Job drawing, mm, ordinate dimensions from the low corner. One solid piece. A direction names the side the tool comes from. Give positions to 0.01 mm unless a question says otherwise; leave off trailing zeros. Order: outer loops, then holes, each group sorted by start corner. A loop starts at its lowest first (then second) coordinate and runs counter-clockwise, first axis right, second up. Notation, with made-up numbers: M 29,-16.75 L 64,-16.75 A9 cw 64,-11.75 Z; hole C 23.25,52.5 d3. An arc over 180 degrees is marked long. One line per item, written item: value. Start each with the question number.
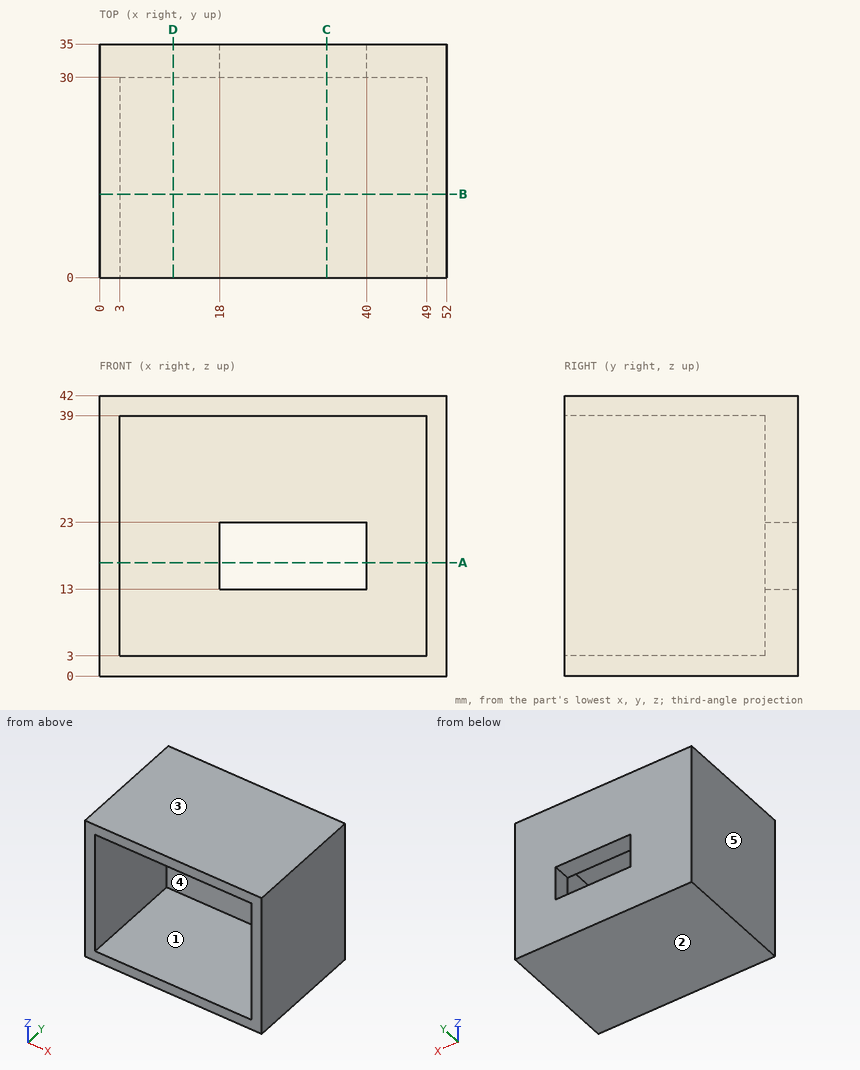
1) Slice it at A-A (z = 17). List the corners of the cut face in (x, y), plus the area to 3 significant figures.
2) Drill centre lines: line 1 (X direction, y = 24, z = 5); line 2 (Z direction, x = 19, y = 29); line 3 (Y direction, x = 45, z = 32.5). Where is each one in solid material? Low to high.
3) Slice it at B-B (y = 12.5). List the corners of the cut face in (x, z), plus the area to 3 significant figures.
4) Slice it at D-D (x = 11). List the corners of the cut face in (y, z), plus the area to 3 significant figures.
5) Drop a flat-ended pin along its axis: P1, Ø2, axis at x = 28, z = 25.5, coming from the -Y side. Give the stop position or say it passes through.
6) Slice it at C-C (x = 34). List the corners of the cut face in (y, z), plus the area to 3 significant figures.
7) Tool access for the marked faces 4 and 5: list every direction of +Z, -Z, +X, -X, +Y, -Y with a clear straight run to the whole face (end or side of a thin tool).
8) Pull direction Z, two halves, no side cores. Call the marked faces 1, 2 and 3: pulls with the +Z half, pulls with the -Z half, needs draft (parallel to the pull), parting line crosses it, or undercut.
Results list:
1. outline: M 0,0 L 3,0 L 3,30 L 18,30 L 18,35 L 0,35 Z; M 40,30 L 49,30 L 49,0 L 52,0 L 52,35 L 40,35 Z
1. area: 330 mm²
2. line 1: x = 0 to 3, 49 to 52
2. line 2: z = 0 to 3, 39 to 42
2. line 3: y = 30 to 35
3. outline: M 0,0 L 52,0 L 52,42 L 0,42 Z; hole M 3,3 L 49,3 L 49,39 L 3,39 Z
3. area: 528 mm²
4. outline: M 0,0 L 35,0 L 35,42 L 0,42 L 0,39 L 30,39 L 30,3 L 0,3 Z
4. area: 390 mm²
5. P1: stops at y = 30
6. outline: M 0,0 L 35,0 L 35,13 L 30,13 L 30,3 L 0,3 Z; M 0,39 L 30,39 L 30,23 L 35,23 L 35,42 L 0,42 Z
6. area: 340 mm²
7. face 4: -Y
7. face 5: +Z, -Z, -X, +Y, -Y
8. face 1: undercut
8. face 2: pulls with the -Z half
8. face 3: pulls with the +Z half
